For this review, take the finished solid that the model builds, in its own axes (mm). Give positions to 0.01 mm unless a question says otherwise; leave off trailing zeros. Order: outer loops, then holes, each group sorted by start corner. A loop starts at its lowest first (then second) coordinate and runs counter-clockwise, first axis right, second up.
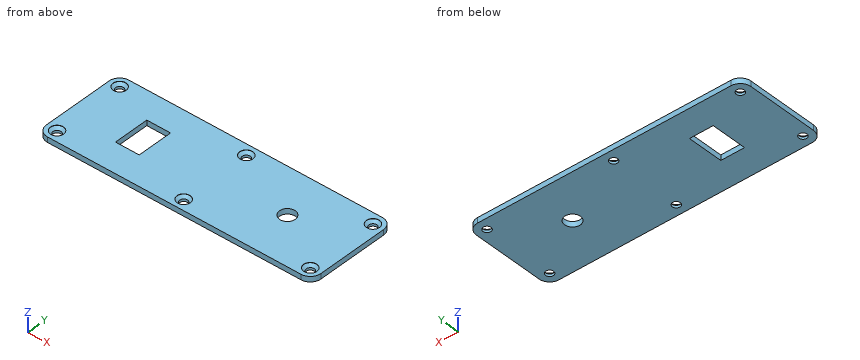
from build123d import *

# Parameters (mm, degrees)
IZIM1_W                     = 104
IZIM1_H                     = 35
Y_KSEKLIK_EKSTR_ZYON1_DEPTH = 2
IZIM2_R                     = 1.5
KES_EKSTR_ZYON1_DEPTH       = 2
IZIM3_R                     = 2.5
KES_EKSTR_ZYON2_DEPTH       = 0.1
PAH2_SIZE                   = 1
IZIM4_R                     = 1.5
KES_EKSTR_ZYON3_DEPTH       = 2
IZIM5_R                     = 2.5
KES_EKSTR_ZYON4_DEPTH       = 0.1
PAH3_SIZE                   = 1
RADYUS1_R                   = 4
IZIM7_R                     = 3
IZIM7_W                     = 9
IZIM7_H                     = 13.5
KES_EKSTR_ZYON6_DEPTH       = 2


with BuildPart() as part:
    # Çizim1 → Yükseklik-Ekstrüzyon1 (new body)
    with BuildSketch(Plane.XY):
        with Locations((-52, 17.5)):
            Rectangle(IZIM1_W, IZIM1_H)
    extrude(amount=Y_KSEKLIK_EKSTR_ZYON1_DEPTH)

    # Çizim2 → Kes-Ekstrüzyon1 (cut)
    with BuildSketch(Plane.XY.offset(2)):
        with Locations((-100, 31)):
            Circle(IZIM2_R)
        with Locations((-100, 4)):
            Circle(IZIM2_R)
        with Locations(Location((-4, 4, 0), (0, 0, 180))):
            Circle(IZIM2_R)
        with Locations(Location((-4, 31, 0), (0, 0, 180))):
            Circle(IZIM2_R)
    extrude(amount=-KES_EKSTR_ZYON1_DEPTH, mode=Mode.SUBTRACT)

    # Çizim3 → Kes-Ekstrüzyon2 (cut)
    with BuildSketch(Plane.XY.offset(2)):
        with Locations((-100, 31)):
            Circle(IZIM3_R)
        with Locations((-100, 4)):
            Circle(IZIM3_R)
        with Locations(Location((-4, 4, 0), (0, 0, 180))):
            Circle(IZIM3_R)
        with Locations(Location((-4, 31, 0), (0, 0, 180))):
            Circle(IZIM3_R)
    extrude(amount=-KES_EKSTR_ZYON2_DEPTH, mode=Mode.SUBTRACT)

    # Pah2
    pah2_edges = [part.edges().sort_by_distance(p)[0] for p in [
        (-2.5, 31, 1.9),
        (-2.5, 4, 1.9),
        (-101.5, 4, 1.9),
        (-101.5, 31, 1.9),
    ]]
    chamfer(pah2_edges, length=PAH2_SIZE - 0.0001)  # a hair under: the kernel refuses the full size

    # Çizim4 → Kes-Ekstrüzyon3 (cut)
    with BuildSketch(Plane.XY.offset(2)):
        with Locations((-52, 31)):
            Circle(IZIM4_R)
        with Locations((-52, 4)):
            Circle(IZIM4_R)
    extrude(amount=-KES_EKSTR_ZYON3_DEPTH, mode=Mode.SUBTRACT)

    # Çizim5 → Kes-Ekstrüzyon4 (cut)
    with BuildSketch(Plane.XY.offset(2)):
        with Locations((-52, 31)):
            Circle(IZIM5_R)
        with Locations((-52, 4)):
            Circle(IZIM5_R)
    extrude(amount=-KES_EKSTR_ZYON4_DEPTH, mode=Mode.SUBTRACT)

    # Pah3
    pah3_edges = [part.edges().sort_by_distance(p)[0] for p in [
        (-53.5, 31, 1.9),
        (-53.5, 4, 1.9),
    ]]
    chamfer(pah3_edges, length=PAH3_SIZE - 0.0001)  # a hair under: the kernel refuses the full size

    # Radyus1
    radyus1_edges = [part.edges().sort_by_distance(p)[0] for p in [
        (0, 0, 1),
        (-104, 0, 1),
        (-104, 35, 1),
        (0, 35, 1),
    ]]
    fillet(radyus1_edges, radius=RADYUS1_R)

    # Çizim7 → Kes-Ekstrüzyon6 (cut)
    with BuildSketch(Plane.XY.offset(2)):
        with Locations((-25, 18)):
            Circle(IZIM7_R)
        with Locations((-79.5, 17.75)):
            Rectangle(IZIM7_W, IZIM7_H)
    extrude(amount=-KES_EKSTR_ZYON6_DEPTH, mode=Mode.SUBTRACT)


solid = part.part
1) Clearance check with flat-ended pins moving along their axes: pin 1 (4 mm diameter, centred on x = -3.5, y = 5, fed in from +Z); pin 2 (2.5 mm diameter, centred on x = -99.5, y = 5, fed in from +Z); pin 3 (1.5 mm diameter, centred on x = -3, y = 30.5, fed in from +Z). State where each tip first meets the part, or that it passes through.
Answer sheet:
pin 1: stops at z = 2
pin 2: stops at z = 1.77
pin 3: stops at z = 1.27
2) We need section D-D on z = 0.5. Count the separate pieces of the cut face and the enclosed holes in it, then the cut area to 3 significant figures.
Answer sheet:
separate pieces: 1
enclosed holes: 8
area: 3,430 mm2
3) We need section C-C on y = 12. Give the boundary of the cut face in (x, z).
Answer sheet:
outline: (-104, 0) - (-84, 0) - (-84, 2) - (-104, 2) - close; (-75, 0) - (0, 0) - (0, 2) - (-75, 2) - close
4) To check wall thickness, follow line 1 (Y direction, x = -52, z = 1.95); line 2 (Y direction, x = -100, z = 0.6); line 3 (X direction, y = 14.5, z = 1.35). State the ranges of each line that lie inside material, in increasing order.
Answer sheet:
line 1: y = 0 to 1.5, 6.5 to 28.5, 33.5 to 35
line 2: y = 0 to 2.5, 5.5 to 29.5, 32.5 to 35
line 3: x = -104 to -84, -75 to 0
5) We need section B-B on y = 18. Give the boundary of the cut face in (x, z), then the cut area to 3 significant figures.
Answer sheet:
outline: (-104, 0) - (-84, 0) - (-84, 2) - (-104, 2) - close; (-75, 0) - (-28, 0) - (-28, 2) - (-75, 2) - close; (-22, 0) - (0, 0) - (0, 2) - (-22, 2) - close
area: 178 mm2
6) We need section A-A on x = -25. Give the boundary of the cut face in (y, z), then the cut area to 3 significant figures.
Answer sheet:
outline: (0, 0) - (15, 0) - (15, 2) - (0, 2) - close; (21, 0) - (35, 0) - (35, 2) - (21, 2) - close
area: 58.0 mm2
